Autodesk Inventor part; units mm, degrees
ref_plane "YZ Plane" through (0, 0, 0) normal (1, 0, 0) x (0, 1, 0)
ref_plane "XZ Plane" through (0, 0, 0) normal (0, 1, 0) x (-1, 0, 0)
ref_plane "XY Plane" through (0, 0, 0) normal (0, 0, 1) x (1, 0, 0)
sketch "Sketch1" plane through (0, 0, 0) normal (0, 1, 0) x (-1, 0, 0)
  line L0 (-2.9, 5.5) -> (2.9, 5.5)
  line L1 (2.9, 5.5) -> (2.9, -5.5)
  line L2 (2.9, -5.5) -> (-2.9, -5.5)
  line L3 (-2.9, -5.5) -> (-2.9, 5.5)
  line L4 (-2.9, 5.5) -> (2.9, -5.5) construction
  line L5 (2.9, 5.5) -> (-2.9, -5.5) construction
  point P0 (0, 0)
  dimension "d0" = 11
  dimension "d1" = 5.8
extrude "Extrusion1" add sketch "Sketch1" along normal mid plane 4.2
sketch "Sketch2" plane through (2.9, -2.1, -5.5) normal (1, 0, 0) x (0, 0, -1)
  line L0 (0, 4.2) -> (0, 0)
  line L1 (-11, 4.2) -> (0, 4.2)
  line L2 (-11, 0) -> (-11, 4.2)
  line L3 (0, 0) -> (-11, 0)
  line L4 (-11, 0) -> (-11, 4.2)
  line L5 (-11, 1.5) -> (-9, 0)
  line L6 (0, 0) -> (-11, 0)
  line L7 (-2, 0) -> (0, 1.5)
  line L8 (-11, 4.2) -> (-8.5, 4.2)
  line L9 (-8.5, 4.2) -> (-8.5, 3.4)
  line L10 (-8.5, 3.4) -> (-11, 3.4)
  line L11 (-11, 3.4) -> (-11, 4.2)
  line L12 (0, 4.2) -> (-2.5, 4.2)
  line L13 (-2.5, 4.2) -> (-2.5, 3.4)
  line L14 (-2.5, 3.4) -> (0, 3.4)
  line L15 (0, 3.4) -> (0, 4.2)
  point P0 (-5.5, 2.1)
  dimension "d4" = 6
  dimension "d5" = 3
  dimension "d6" = 7
  dimension "d7" = 3.5
  dimension "d8" = 1.5
  dimension "d9" = 3.4
extrude "Extrusion2" cut sketch "Sketch2" against normal through all contours L0 L14 L13 L1 | L0 L3 L7 | L9 L10 L2 L1 | L3 L2 L5
sketch "Sketch3" plane through (0, 2.1, 0) normal (0, 1, 0) x (1, 0, 0)
  point P0 (0, 0)
  point P1 (0, 0)
hole "Hole1" at (0, 2.1, 0) direction (0, -1, 0) diameter 3.242 end through all
properties part number "RHOMBUS NUT 4"
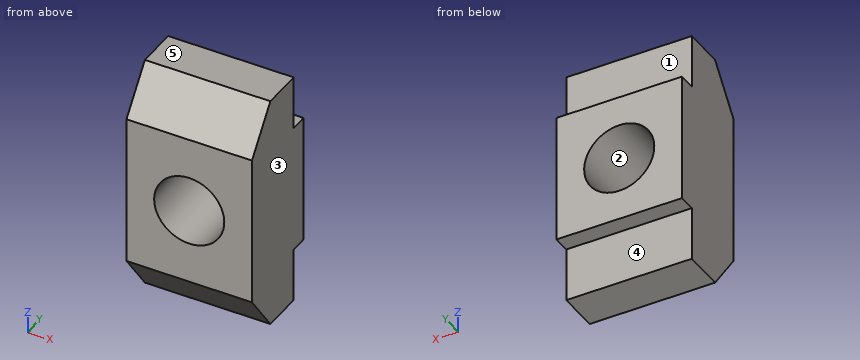
Design review of the part built by this model. Coordinates are the model's own, in mm. Face numbers are marked on the shaded views. A direction names the side the tool comes from. Round coordinates to 2 decimals unless told otherwise and drop trailing zeros. Order: outer loops, then holes, each group sorted by start corner. A loop starts at its lowest first (then second) coordinate and runs counter-clockwise, first axis right, second up.
1) Draft analysis for pull direction X (two halves, no side actions). For the marked faces 1, 2 and 3, state which applies: released by +X, released by -X, zero draft, split by the parting line, or undercut.
The answers:
face 1: zero draft
face 2: undercut
face 3: released by +X
2) Consider section B-B (z = 0). State the section outline as (x, y) points, plus the area to 3 significant figures.
The answers:
outline: (-2.9, -2.1) - (-1.62, -2.1) - (-1.62, 2.1) - (-2.9, 2.1) - close; (1.62, -2.1) - (2.9, -2.1) - (2.9, 2.1) - (1.62, 2.1) - close
area: 10.7 mm2
3) Machinability: for the marked faces 4 and 5, which of the approach directions +Z, -Z, +X, -X, +Y, -Y give a long, thin tool a straight path to every point of the face, cutting with its end or side? Answer none if there is none.
The answers:
face 4: -Z, +X, -X, +Y
face 5: +Z, +X, -X, +Y, -Y
4) Consider section C-C (y = 0.4). State the section outline as (x, z) points, plus the area to 3 significant figures.
The answers:
outline: (-2.9, -5.5) - (2.9, -5.5) - (2.9, 5.5) - (-2.9, 5.5) - close; hole circle Ø3.24 at (0, 0)
area: 55.5 mm2
5) For L1, parallel to Z at x = 0, y = -0.3; L2, parallel to X at y = -0.9, z = 0; L3, parallel to X at y = -0.05, z = -0.5, list the stretches that pass through material, from the lowest coordinate up.
The answers:
L1: z = -5.5 to -1.62, 1.62 to 5.5
L2: x = -2.9 to -1.62, 1.62 to 2.9
L3: x = -2.9 to -1.54, 1.54 to 2.9
6) Consider section D-D (x = -1.95). State the section outline as (y, z) points.
The answers:
outline: (-2.1, -3.5) - (-0.6, -5.5) - (1.3, -5.5) - (1.3, -3) - (2.1, -3) - (2.1, 3) - (1.3, 3) - (1.3, 5.5) - (-0.6, 5.5) - (-2.1, 3.5) - close
7) Clearance check with flat-ended pins moving along their axes: pin 1 Ø1.2 at (x, z) = (1.5, 4) entering from +Y; pin 2 Ø0.9 at (x, y) = (-1.5, 1.5) entering from +Z; pin 3 Ø3 at (x, z) = (0, 0) entering from -Y. State where each tip first meets the part, or that it passes through.
The answers:
pin 1: stops at y = 1.3
pin 2: stops at z = 5.5
pin 3: passes through
8) Consider section A-A (x = 0). State the section outline as (y, z) points.
The answers:
outline: (-2.1, -3.5) - (-0.6, -5.5) - (1.3, -5.5) - (1.3, -3) - (2.1, -3) - (2.1, -1.62) - (-2.1, -1.62) - close; (-2.1, 1.62) - (2.1, 1.62) - (2.1, 3) - (1.3, 3) - (1.3, 5.5) - (-0.6, 5.5) - (-2.1, 3.5) - close
